The listing builds one solid part. Answer for the finished solid, in the listing's coordinates (mm). A direction names the side the tool comes from. Give positions to 0.01 mm unless a question says otherwise; leave off trailing zeros. Order: outer loops, then holes, each group sorted by start corner. A loop starts at its lowest first (then second) coordinate and runs counter-clockwise, first axis right, second up. Notation, with made-up numbers: (33.5, 3) - (70.5, 3) arc R9 cw to (70.5, 10) - close; hole circle Ø1 at (38.5, -15.5). An arc over 180 degrees is marked (long way). Use a Markdown table: item, result. Add a question column.
1) Find section A-A, the plane y = -6. Determine the outline of the cut face in (x, z).
2) Straight lines are drawn through the part: line 1 (Y direction, x = 55, z = 0.95); line 2 (X direction, y = 87.1, z = 0.9); line 3 (X direction, y = -7.5, z = 0.9). For each, find the intervals that lie inside material, in ascending order.
3) Find section B-B, the plane z = 1. Determine the outline of the cut face in (x, y), plus the area to 3 significant figures.
4) Flat-ended cylindrical pins translate along their axes: pin 1 (0.8 mm diameter, centred on x = 64.5, z = 1.5, fed in from -Y); pin 2 (0.6 mm diameter, centred on y = 14.5, z = 0.5, fed in from -X); pin 3 (0.6 mm diameter, centred on y = -6, z = 0.5, fed in from +X). Find the tip coordinate at first contact, or state that the pin passes through.
5) Find section C-C, the plane x = 39. Determine the outline of the cut face in (y, z), plus the area to 3 significant figures.
6) The mould has two halves that part along X. Classify faces 4 (the face through (52, 0, 1)), 5 (the face through (46, -15, 1)), 6 (the face through (0, 78, 1)): released by +X, released by -X, zero draft, split by the parting line, or undercut.
7) Find section D-D, the plane y = 28.5. Determine the outline of the cut face in (x, z), plus the area to 3 significant figures.
8) For faces 1 (the face through (53.5, -8, 1)), 2 (the face through (63.5, -7, 1)), 3 (the face through (39, 0, 1)), determine the directions among +Z, -Z, +X, -X, +Y, -Y from which every point of the face is accessible in a straight line to the end or side of a thin tool.
Autodesk Inventor part; units mm, degrees
ref_plane "YZ Plane" through (0, 0, 0) normal (1, 0, 0) x (0, 1, 0)
ref_plane "XZ Plane" through (0, 0, 0) normal (0, 1, 0) x (-1, 0, 0)
ref_plane "XY Plane" through (0, 0, 0) normal (0, 0, 1) x (1, 0, 0)
sketch "Sketch4" plane through (0, 0, 0) normal (0, 0, 1) x (1, 0, 0)
  line L0 (0, 0) -> (65, 0)
  line L1 (65, 0) -> (65, 100)
  line L2 (65, 100) -> (0, 100)
  line L3 (0, 100) -> (0, 0)
  line L4 (1.5, 0) -> (11.5, 0)
  line L5 (11.5, 0) -> (11.5, -15)
  line L6 (11.5, -15) -> (1.5, -15)
  line L7 (1.5, -15) -> (1.5, 0)
  line L8 (14.5, 0) -> (24.5, 0)
  line L9 (24.5, 0) -> (24.5, -15)
  line L10 (24.5, -15) -> (14.5, -15)
  line L11 (14.5, -15) -> (14.5, 0)
  line L12 (32.5, 0) -> (42.5, 0)
  line L13 (27.5, 0) -> (37.5, 0)
  line L14 (37.5, 0) -> (37.5, -15)
  line L15 (37.5, -15) -> (27.5, -15)
  line L16 (27.5, -15) -> (27.5, 0)
  line L17 (40.5, 0) -> (50.5, 0)
  line L18 (50.5, 0) -> (50.5, -15)
  line L19 (50.5, -15) -> (40.5, -15)
  line L20 (40.5, -15) -> (40.5, 0)
  line L21 (53.5, 0) -> (63.5, 0)
  line L22 (63.5, 0) -> (63.5, -15)
  line L23 (63.5, -15) -> (53.5, -15)
  line L24 (53.5, -15) -> (53.5, 0)
  dimension "d39" = 65
  dimension "d40" = 100
  dimension "d41" = 10
  dimension "d42" = 15
  dimension "d43" = 1.5
  dimension "d44" = 10
  dimension "d45" = 15
  dimension "d47" = 3
  dimension "d49" = 10
  dimension "d50" = 10
  dimension "d51" = 15
  dimension "d52" = 3
  dimension "d53" = 3
  dimension "d54" = 10
  dimension "d55" = 15
  dimension "d56" = 3
extrude "Extrusion4" add sketch "Sketch4" along normal blind 2
sketch "Sketch5" plane through (0, 0, 2) normal (0, 0, 1) x (1, 0, 0)
  circle A0 centre (55, 80) radius 0.75
  line L0 (65, 100) -> (0, 100)
  line L1 (65, 0) -> (65, 100)
  circle A1 centre (55, 72.9) radius 0.75
  circle A2 centre (55, 87.1) radius 0.75
  point P0 (0, 0)
  dimension "d59" = 1.5
  dimension "d60" = 20
  dimension "d61" = 10
  dimension "d62" = 1.5
  dimension "d63" = 7.1
  dimension "d64" = 1.5
  dimension "d65" = 7.1
extrude "Extrusion5" cut sketch "Sketch5" against normal blind 2
sketch "Sketch6" plane through (0, 0, 2) normal (0, 0, 1) x (1, 0, 0)
  line L0 (0, -15) -> (37.5, -15)
  line L1 (37.5, -15) -> (37.5, 55)
  line L2 (37.5, 55) -> (0, 55)
  line L3 (0, 55) -> (0, -15)
  point P0 (0, 0)
  dimension "d68" = 37.5
  dimension "d69" = 70
extrude "Extrusion6" cut sketch "Sketch6" against normal blind 2
properties part number "Arm"
The answers:
| question | item | result |
|---|---|---|
| 1 | outline | (40.5, 0) - (50.5, 0) - (50.5, 2) - (40.5, 2) - close; (53.5, 0) - (63.5, 0) - (63.5, 2) - (53.5, 2) - close |
| 2 | line 1 | -15 to 72.15, 73.65 to 79.25, 80.75 to 86.35, 87.85 to 100 |
| 2 | line 2 | 0 to 54.25, 55.75 to 65 |
| 2 | line 3 | 40.5 to 50.5, 53.5 to 63.5 |
| 3 | outline | (0, 55) - (37.5, 55) - (37.5, 0) - (40.5, 0) - (40.5, -15) - (50.5, -15) - (50.5, 0) - (53.5, 0) - (53.5, -15) - (63.5, -15) - (63.5, 0) - (65, 0) - (65, 100) - (0, 100) - close; hole circle Ø1.5 at (55, 72.9); hole circle Ø1.5 at (55, 80); hole circle Ø1.5 at (55, 87.1) |
| 3 | area | 4,730 mm2 |
| 4 | pin 1 | y = 0 |
| 4 | pin 2 | x = 37.5 |
| 4 | pin 3 | x = 63.5 |
| 5 | outline | (0, 0) - (100, 0) - (100, 2) - (0, 2) - close |
| 5 | area | 200 mm2 |
| 6 | face 4 | undercut |
| 6 | face 5 | zero draft |
| 6 | face 6 | released by -X |
| 7 | outline | (37.5, 0) - (65, 0) - (65, 2) - (37.5, 2) - close |
| 7 | area | 55.0 mm2 |
| 8 | face 1 | +Z, -Z, -Y |
| 8 | face 2 | +Z, -Z, +X, -Y |
| 8 | face 3 | +Z, -Z, -X, -Y |
